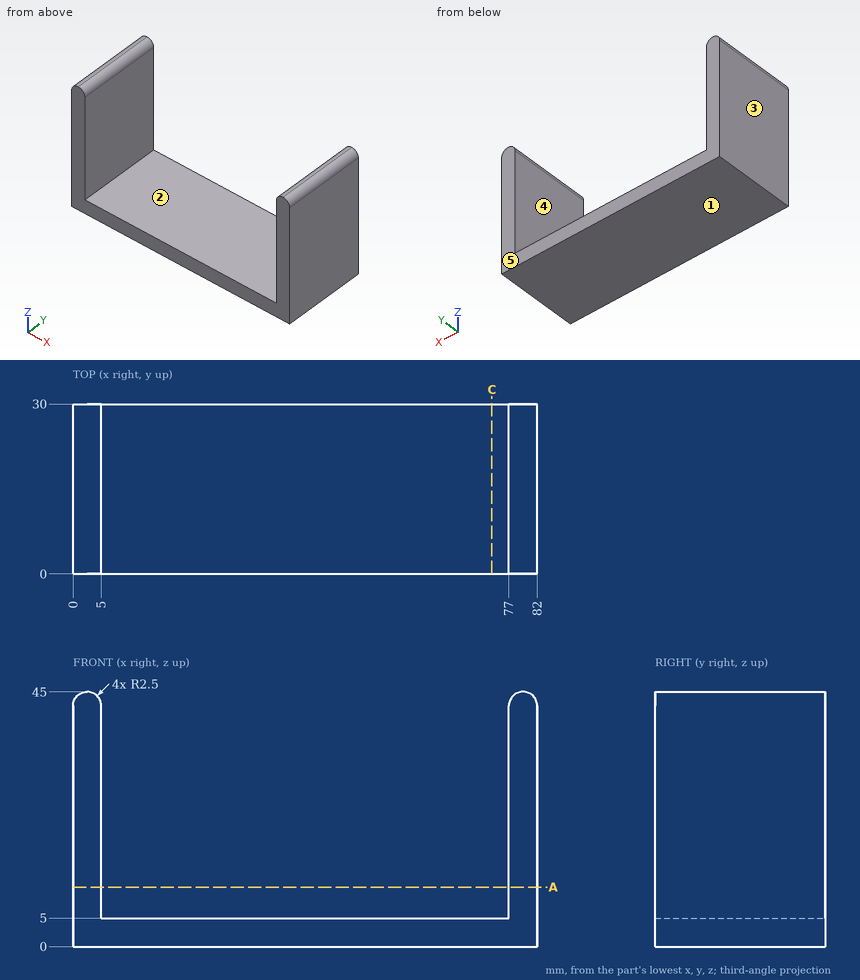
Verification items for this drawing (mm, ordinates from the low corner). A direction names the side the tool comes from. Round coordinates to 2 decimals unless told otherwise and drop trailing zeros. Order: outer loops, then holes, each group sorted by start corner. A loop starts at its lowest first (then second) coordinate and runs counter-clockwise, first axis right, second up. Notation, with made-up numbers: (-26.75, 54.5) -> (30.25, 54.5) arc R29 ccw to (30.25, 76.5) -> close; hole circle Ø7 at (15.5, 37). An arc over 180 degrees is marked (long way). Use one line per item in the form item = value.
1. Cross-section at C-C, the plane x = 74. Enter the section's corners in (y, z), plus the area to 3 significant figures.
Working result:
outline = (0, 0) -> (30, 0) -> (30, 5) -> (0, 5) -> close
area = 150 mm^2
2. Cross-section at A-A, the plane z = 10.5. Enter the section's corners in (x, y), plus the area to 3 significant figures.
Working result:
outline = (0, 0) -> (5, 0) -> (5, 30) -> (0, 30) -> close; (77, 0) -> (82, 0) -> (82, 30) -> (77, 30) -> close
area = 300 mm^2
3. Set-up check for the marked faces 4 and 5: record each of +Z, -Z, +X, -X, +Y, -Y from which the full face is reachable in a straight line by a thin tool's end or side.
Working result:
face_4 = +Z, +Y, -Y
face_5 = +Z, -Z, +X, -X, +Y
4. Mould release check, pull along X, two halves, no side actions. Record for the marked faces 1, 2 and 3: pulls with the +X half, pulls with the -X half, needs draft (parallel to the pull), parting line crosses it, or undercut.
Working result:
face_1 = needs draft
face_2 = undercut
face_3 = pulls with the -X half
5. Scan lines: line 1 along X through (y, z) = (11.25, 11); line 2 along Z through (x, y) = (13, 7.5). Record each from-to range of solid material in increasing order. Write a range as from..to.
Working result:
line_1 = 0..5, 77..82
line_2 = 0..5
6. Go/stop test with flat-tipped pins: pin 1 (12 mm diameter, centred on x = 18, z = 14.5, fed in from -Y); pin 2 (5 mm diameter, centred on x = 63, y = 20, fed in from +Z). Record where each tip stops, or that it passes through.
Working result:
pin_1 = through
pin_2 = 5
